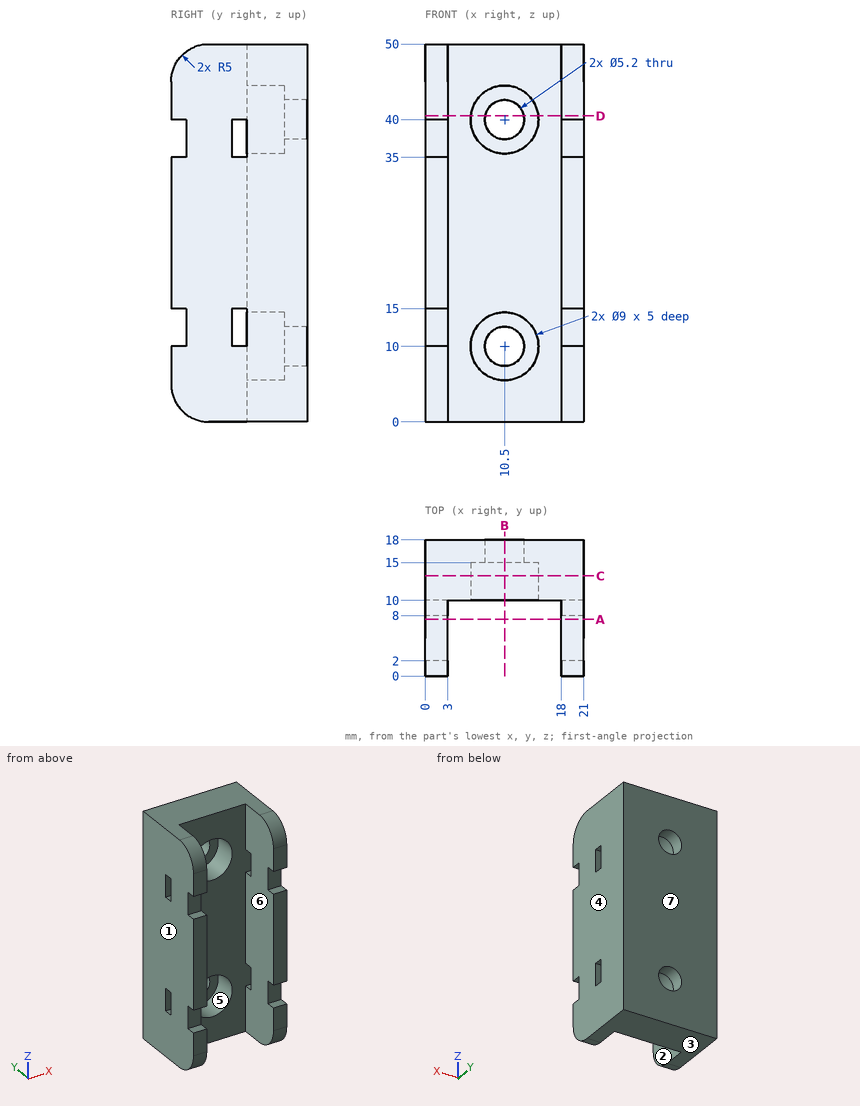
Design review of the part shown in the three views and the two pictorial views. Dimensions are in mm from the part's minimum x, y and z. A direction names the side the tool comes from. Coordinates: 2 decimals unless noted, no trailing zeros. Write each loop counter-clockwise with the first axis right and the second up, starting at its lowest first coordinate (ties: lowest second). Pieces come first, ordered by that corner, then holes.
(1) Add section C-C on y = 13.25. Give the boundary of the cut face in (x, z).
(2) For pin 1 Ø0.6 at (x, y) = (19, 1) entering from +Z; pin 2 Ø10.5 at (x, z) = (10.5, 40) entering from -Y; pin 3 Ø0.6 at (x, y) = (2, 0.5) entering from -Z, all flat-tipped, find the tip position at first contact; note any pin that passes through.
(3) Add section B-B on x = 10.5. Give the boundary of the cut face in (y, z).
(4) Tool access review of the marked faces 5, 6 and 7: name each direction out of +Z, -Z, +X, -X, +Y, -Y from which nothing blocks a thin tool from reaching the whole face with its end or side.
(5) Add section D-D on z = 40.5. Give the boundary of the cut face in (x, y), then the cut area to 3 significant figures.
(6) Wall thickness on probe 1 along Z at (x, y) = (2.5, 9.5); probe 2 along Z at (x, y) = (10.5, 11.2); probe 3 along X at (y, z) = (12.55, 40): over which ranges is each line inside the solid? List them lowest first.
(7) Add section A-A on y = 7.5. Give the boundary of the cut face in (x, z), then the cut area to 3 significant figures.
(8) The part is to be moulded in two halves that separate along X. For the marked faces 1, 2, 3 and 4, say which applies: +X half, -X half, draft (parallel to the pull), parting line (faces both ways), or undercut.
Answer sheet:
1. outline: (0, 0) - (21, 0) - (21, 50) - (0, 50) - close; hole circle Ø9 at (10.5, 10); hole circle Ø9 at (10.5, 40)
2. pin 1: stops at z = 48.36
2. pin 2: stops at y = 10
2. pin 3: stops at z = 2.29
3. outline: (10, 0) - (18, 0) - (18, 7.4) - (15, 7.4) - (15, 5.5) - (10, 5.5) - close; (10, 14.5) - (15, 14.5) - (15, 12.6) - (18, 12.6) - (18, 37.4) - (15, 37.4) - (15, 35.5) - (10, 35.5) - close; (10, 44.5) - (15, 44.5) - (15, 42.6) - (18, 42.6) - (18, 50) - (10, 50) - close
4. face 5: -Y
4. face 6: +Z, -Z, -Y
4. face 7: +Z, -Z, +X, -X, +Y
5. outline: (0, 0) - (3, 0) - (3, 10) - (6.03, 10) - (6.03, 15) - (7.95, 15) - (7.95, 18) - (0, 18) - close; (13.05, 15) - (14.97, 15) - (14.97, 10) - (18, 10) - (18, 0) - (21, 0) - (21, 18) - (13.05, 18) - close
5. area: 168 mm2
6. probe 1: z = 0 to 10, 15 to 35, 40 to 50
6. probe 2: z = 0 to 5.5, 14.5 to 35.5, 44.5 to 50
6. probe 3: x = 0 to 6, 15 to 21
7. outline: (0, 0) - (3, 0) - (3, 50) - (0, 50) - close; (18, 0) - (21, 0) - (21, 50) - (18, 50) - close
7. area: 300 mm2
8. face 1: -X half
8. face 2: undercut
8. face 3: draft
8. face 4: +X half
